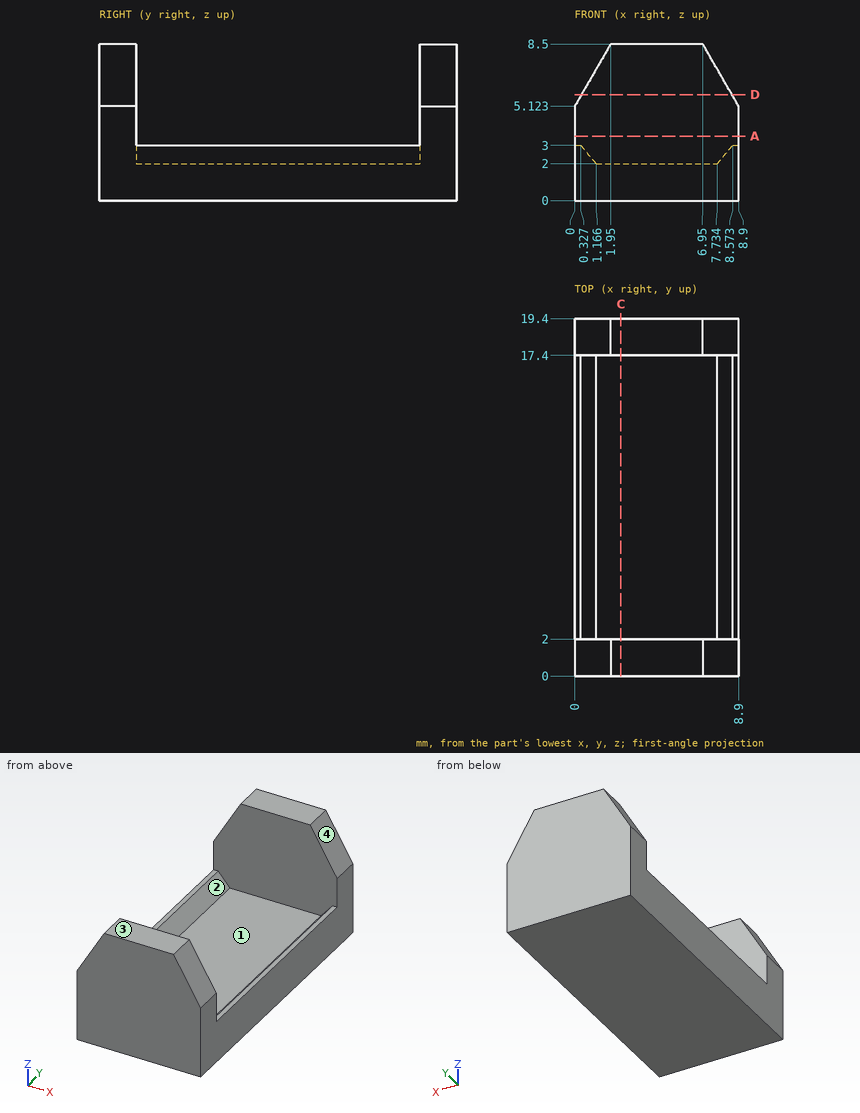
Print and shaded views of the part. All mm, measured from the part's lowest x, y and z. Round coordinates to 2 decimals unless told otherwise and drop trailing zeros. Order: outer loops, then holes, each group sorted by start corner. A loop starts at its lowest first (then second) coordinate and runs counter-clockwise, first axis right, second up.
Q1. Slice it at A-A (z = 3.5). Write the cut outline in (x, y).
Q2. Slice it at D-D (z = 5.75). Write the cut outline in (x, y), and give its area (3 significant figures).
Q3. Two-plate mould, pull along X, no slides. Class the marked faces 1, 2, 3 and 4: pulls with the +X half, pulls with the -X half, needs draft (parallel to the pull), parting line crosses it, or undercut.
Q4. Wall check: L1, parallel to Y at x = 4.5, z = 7; L2, parallel to Z at x = 2.25, y = 5.25; L3, parallel to Z at x = 8, y = 11 (1 decimal). Give the ranges that are in metal, low to high.
Q5. Slice it at C-C (x = 2.5). Write the cut outline in (y, z).
Results below:
1. outline: (0, 0) - (8.9, 0) - (8.9, 2) - (0, 2) - close; (0, 17.4) - (8.9, 17.4) - (8.9, 19.4) - (0, 19.4) - close
2. outline: (0.36, 0) - (8.54, 0) - (8.54, 2) - (0.36, 2) - close; (0.36, 17.4) - (8.54, 17.4) - (8.54, 19.4) - (0.36, 19.4) - close
2. area: 32.7 mm2
3. face 1: undercut
3. face 2: undercut
3. face 3: needs draft
3. face 4: pulls with the +X half
4. L1: y = 0 to 2, 17.4 to 19.4
4. L2: z = 0 to 2
4. L3: z = 0 to 2.3
5. outline: (0, 0) - (19.4, 0) - (19.4, 8.5) - (17.4, 8.5) - (17.4, 2) - (2, 2) - (2, 8.5) - (0, 8.5) - close
